from build123d import *

# Parameters (mm, degrees)
HITCH_PROFILE_FOR_EXTRUSION_DEPTH = 31.75
SKETCH2_R                         = 9.525
BALL_ANCHOR_HOLE_DEPTH            = 77.2
F_45_DEG_CORNERS_DEPTH            = 77.2
BOLT_HOLE_X_2_REACH               = 17.875
SKETCH4_R                         = 6.35


with BuildPart() as part:
    # Sketch1 → Hitch Profile for Extrusion (new body, symmetric)
    with BuildSketch(Plane.XY):
        with BuildLine():
            Line((-76.2, -60.325), (-76.2, -19.05))
            ThreePointArc((-76.2, -19.05), (-65.970704333, 5.645704333), (-41.275, 15.875))
            Line((-41.275, 15.875), (25.4, 15.875))
            Line((25.4, 15.875), (25.4, 0))
            Line((25.4, 0), (-41.275, 0))
            ThreePointArc((-41.275, 0), (-54.745384182, -5.579615818), (-60.325, -19.05))
            Line((-60.325, -19.05), (-60.325, -60.325))
            Line((-60.325, -60.325), (-76.2, -60.325))
        make_face()
    extrude(amount=HITCH_PROFILE_FOR_EXTRUSION_DEPTH, both=True)

    # Sketch2 → Ball Anchor hole (cut, through all)
    with BuildSketch(Plane(origin=(0, 15.875, 0), x_dir=(1, 0, 0), z_dir=(0, 1, 0))):
        Circle(SKETCH2_R)
    extrude(amount=-BALL_ANCHOR_HOLE_DEPTH, mode=Mode.SUBTRACT)

    # Sketch3 → 45 Deg Corners (cut, through all)
    with BuildSketch(Plane(origin=(0, 15.875, 0), x_dir=(1, 0, 0), z_dir=(0, 1, 0))):
        Polygon((12.7, 31.75), (25.4, 19.05), (25.4, 31.75), align=None)
        Polygon((12.7, -31.75), (25.4, -19.05), (25.4, -31.75), align=None)
    extrude(amount=-F_45_DEG_CORNERS_DEPTH, mode=Mode.SUBTRACT)

    # Sketch4 → Bolt Hole x 2 (cut, up to next)
    with BuildSketch(Plane(origin=(-60.325, 0, 0), x_dir=(0, 0, -1), z_dir=(1, 0, 0)), mode=Mode.PRIVATE) as bolt_hole_x_2_sk1:
        with Locations((-15.875, -34.925)):
            Circle(SKETCH4_R)
    bolt_hole_x_2_tool1 = extrude(bolt_hole_x_2_sk1.sketch, amount=-BOLT_HOLE_X_2_REACH, mode=Mode.PRIVATE) & part.part
    add(bolt_hole_x_2_tool1.solids().sort_by_distance((-60.325, -34.925, 15.875))[0], mode=Mode.SUBTRACT)
    # Sketch4 → Bolt Hole x 2 (cut, up to next)
    with BuildSketch(Plane(origin=(-60.325, 0, 0), x_dir=(0, 0, -1), z_dir=(1, 0, 0)), mode=Mode.PRIVATE) as bolt_hole_x_2_sk2:
        with Locations((15.875, -34.925)):
            Circle(SKETCH4_R)
    bolt_hole_x_2_tool2 = extrude(bolt_hole_x_2_sk2.sketch, amount=-BOLT_HOLE_X_2_REACH, mode=Mode.PRIVATE) & part.part
    add(bolt_hole_x_2_tool2.solids().sort_by_distance((-60.325, -34.925, -15.875))[0], mode=Mode.SUBTRACT)


solid = part.part
Check sheet for the modelled part. Datum: model origin and axes. Units: mm. A direction names the side the tool comes from. Coordinates: 2 decimals unless noted, no trailing zeros. Loops run counter-clockwise (first coordinate to the right, second up) from the corner with the lowest first, then second, coordinate; pieces in that order, holes last. Notation, with made-up numbers: (39, -12.75) -> (59, -12.75) arc R21 cw to (59, -8.75) -> close; hole circle Ø6 at (76.5, 27). An arc over 180 degrees is marked (long way). Answer in a Markdown table with one row per item.
1. Material ranges on line 1 along Z through (x, y) = (0, 11.5) (3 decimals); line 2 along X through (y, z) = (-40.5, 9.5) (3 decimals); line 3 along Y through (x, z) = (21.5, -20.5) (3 decimals), recorded low to high. Write a range as [from, to].
Check values:
| item | result |
|---|---|
| line 1 | z = [-31.75, -9.525], [9.525, 31.75] |
| line 2 | x = [-76.2, -60.325] |
| line 3 | y = [0, 15.875] |
2. Sectioned sample at D-D, the plane x = -62. Record the boundary of the cut face in (y, z) (3 decimals).
Check values:
| item | result |
|---|---|
| outline | (-60.325, -31.75) -> (9.061, -31.75) -> (9.061, 31.75) -> (-60.325, 31.75) -> close; hole circle Ø12.7 at (-34.925, -15.875); hole circle Ø12.7 at (-34.925, 15.875) |
3. Sectioned sample at A-A, the plane z = 0. Record the boundary of the cut face in (x, y) (3 decimals), then the cut area to 3 significant figures.
Check values:
| item | result |
|---|---|
| outline | (-76.2, -60.325) -> (-60.325, -60.325) -> (-60.325, -19.05) arc R19.05 cw to (-41.275, 0) -> (-9.525, 0) -> (-9.525, 15.875) -> (-41.275, 15.875) arc R34.925 ccw to (-76.2, -19.05) -> close; (9.525, 0) -> (25.4, 0) -> (25.4, 15.875) -> (9.525, 15.875) -> close |
| area | 2,080 mm2 |
4. Release check for a two-part mould opening along Y. For faces 3 (the face through (-68, -60.325, 0)), 4 (the face through (-66.241, 5.373, 0.444)), 5 (the face through (18.96, 8.05, 25.49)), 6 (the face through (-68.151, -41.124, 17.252)) record: released by +Y, released by -Y, zero draft, split by the parting line, or undercut.
Check values:
| item | result |
|---|---|
| face 3 | released by -Y |
| face 4 | released by +Y |
| face 5 | zero draft |
| face 6 | undercut |
5. Sectioned sample at B-B, the plane x = 0. Record the boundary of the cut face in (y, z) (3 decimals), then the cut area to 3 significant figures.
Check values:
| item | result |
|---|---|
| outline | (0, -31.75) -> (15.875, -31.75) -> (15.875, -9.525) -> (0, -9.525) -> close; (0, 9.525) -> (15.875, 9.525) -> (15.875, 31.75) -> (0, 31.75) -> close |
| area | 706 mm2 |
6. Sectioned sample at C-C, the plane y = -40. Record the boundary of the cut face in (x, z) (3 decimals), then the cut area to 3 significant figures.
Check values:
| item | result |
|---|---|
| outline | (-76.2, -31.75) -> (-60.325, -31.75) -> (-60.325, -19.692) -> (-76.2, -19.692) -> close; (-76.2, -12.058) -> (-60.325, -12.058) -> (-60.325, 12.058) -> (-76.2, 12.058) -> close; (-76.2, 19.692) -> (-60.325, 19.692) -> (-60.325, 31.75) -> (-76.2, 31.75) -> close |
| area | 766 mm2 |
7. Go/stop test with flat-tipped pins: pin 1 (5 mm diameter, centred on x = -44, z = 7, fed in from +Y); pin 2 (3 mm diameter, centred on y = -41.5, z = 6, fed in from +X) (3 decimals); pin 3 (5 mm diameter, centred on x = -52, z = 22.5, fed in from -Y); pin 4 (10 mm diameter, centred on y = -34.925, z = 15.875, fed in from -X). Record where each tip stops, or that it passes through.
Check values:
| item | result |
|---|---|
| pin 1 | stops at y = 15.87 |
| pin 2 | stops at x = -60.325 |
| pin 3 | stops at y = -5.34 |
| pin 4 | passes through |
8. Access from +Z, -Z, +X, -X, +Y, -Y to the whole of each face (thin tool, end or side, straight path). Record for faces 1 (the face through (-60.325, -39, 0)), 2 (the face through (-41, 1, -31.75)).
Check values:
| item | result |
|---|---|
| face 1 | +Z, -Z, +X, -Y |
| face 2 | -Z, +X, -X, +Y, -Y |
